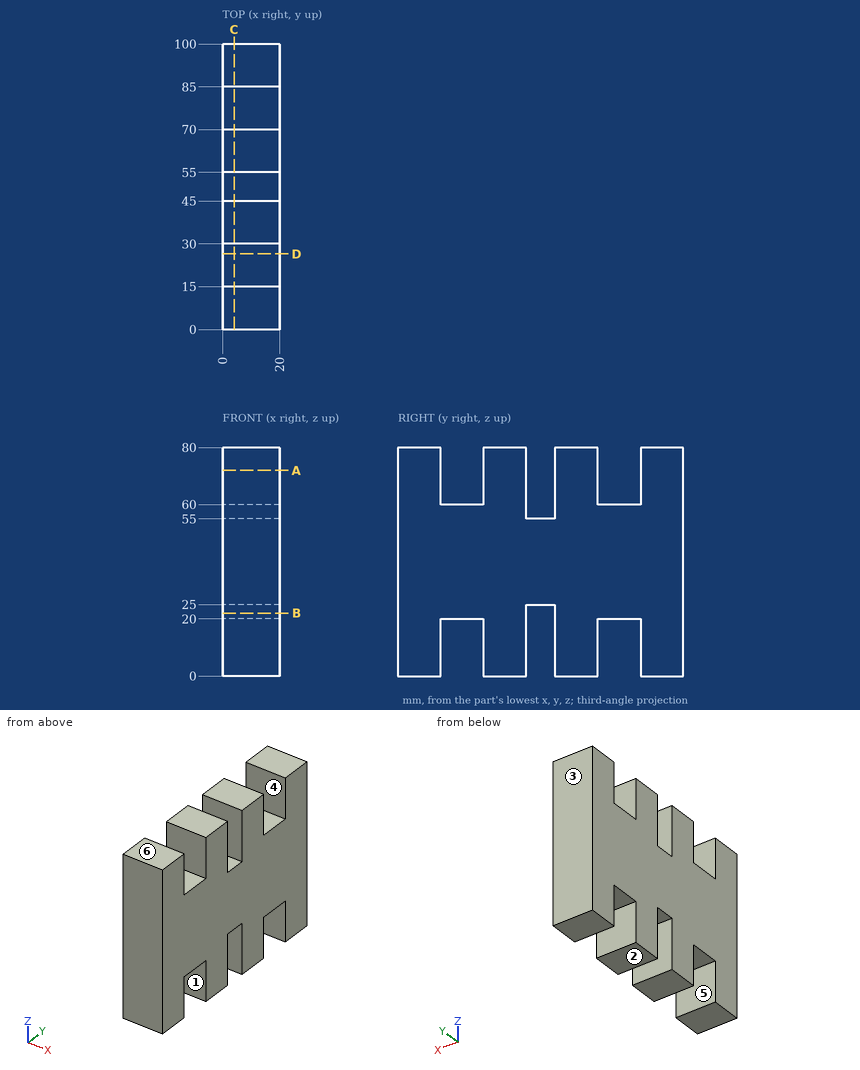
Source: three-view drawing plus pictorial views. Frame: mm from the lowest corner of the part. A direction names the side the tool comes from. Give positions to 0.01 mm unless a question says otherwise; leave off trailing zeros. Write each loop counter-clockwise with the first axis right and the second up, starting at its lowest first coordinate (ties: lowest second). Pieces come first, ordered by that corner, then holes. Notation, with made-up numbers: (-11.5, -36) - (46.5, -36) arc R33 cw to (46.5, -6) - close; hole circle Ø3 at (-38.5, -25.75). An arc over 180 degrees is marked (long way). Write item = value, one per line. Start each with the question number.
1. Mould query, pull axis Y, two halves, no side actions, for the marked faces 1, 2 and 3. Classes: released by +Y, released by -Y, zero draft, split by the parting line, or undercut.
2. Section query D-D, the plane y = 26.5. Output: boundary loops of the cut face in (x, z), then the cut area to 3 significant figures.
3. Section query C-C, the plane x = 4. Output: boundary loops of the cut face in (y, z).
4. Section query B-B, the plane z = 22. Output: boundary loops of the cut face in (x, y).
5. Section query A-A, the plane z = 72. Output: boundary loops of the cut face in (x, y), then the cut area to 3 significant figures.
6. Ray query, L1, parallel to Y at x = 12, z = 62; L2, parallel to Y at x = 5, z = 57; L3, parallel to Z at x = 3.5, y = 72. Return the intervals inside material, ascending.
7. First-contact query: pin 1 Ø4.5 at (x, y) = (8.5, 77) entering from -Z. Flat tip, straight axial feed; report the tip coordinate or a pass-through.
8. Access query for the marked faces 4, 5 and 6. Directions: +Z, -Z, +X, -X, +Y, -Y. A direction counts if a zero-diameter tool reaches every point of the face in a straight line with its end or side. Return the directions, or none.
Check sheet entries:
q1.face_1 = undercut
q1.face_2 = zero draft
q1.face_3 = released by +Y
q2.outline = (0, 20) - (20, 20) - (20, 60) - (0, 60) - close
q2.area = 800 mm2
q3.outline = (0, 0) - (15, 0) - (15, 20) - (30, 20) - (30, 0) - (45, 0) - (45, 25) - (55, 25) - (55, 0) - (70, 0) - (70, 20) - (85, 20) - (85, 0) - (100, 0) - (100, 80) - (85, 80) - (85, 60) - (70, 60) - (70, 80) - (55, 80) - (55, 55) - (45, 55) - (45, 80) - (30, 80) - (30, 60) - (15, 60) - (15, 80) - (0, 80) - close
q4.outline = (0, 0) - (20, 0) - (20, 45) - (0, 45) - close; (0, 55) - (20, 55) - (20, 100) - (0, 100) - close
q5.outline = (0, 0) - (20, 0) - (20, 15) - (0, 15) - close; (0, 30) - (20, 30) - (20, 45) - (0, 45) - close; (0, 55) - (20, 55) - (20, 70) - (0, 70) - close; (0, 85) - (20, 85) - (20, 100) - (0, 100) - close
q5.area = 1,200 mm2
q6.L1 = 0 to 15, 30 to 45, 55 to 70, 85 to 100
q6.L2 = 0 to 45, 55 to 100
q6.L3 = 20 to 60
q7.pin_1 = 20
q8.face_4 = +Z, +X, -X
q8.face_5 = -Z, +X, -X
q8.face_6 = +Z, +X, -X, +Y, -Y
